from build123d import *

# Parameters (mm, degrees)
ESQUISSE1_R        = 2
ESQUISSE1_W        = 5
ESQUISSE1_H        = 10
BOSS_EXTRU_1_DEPTH = 6


with BuildPart() as part:
    # Esquisse1 → Boss.-Extru.1 (new body)
    with BuildSketch(Plane.XY):
        Polygon((0, 0), (0, 26), (-5.2, 26), (-5.2, 20), (-10, 20), (-10, 26), (-15.2, 26), (-15.2, 20), (-20, 20), (-20, 26), (-25.2, 26), (-25.2, 20), (-30, 20), (-30, 26), (-35.2, 26), (-35.2, 20), (-40, 20), (-40, 26), (-45.2, 26), (-45.2, 20), (-50, 20), (-50, 26), (-55.2, 26), (-55.2, 20), (-60, 20), (-60, 26), (-65.2, 26), (-65.2, 20), (-70, 20), (-70, 26), (-75.2, 26), (-75.2, 20), (-80, 20), (-80, 26), (-85.2, 26), (-85.2, 20), (-90, 20), (-90, 26), (-95.2, 26), (-95.2, 20), (-100, 20), (-100, 26), (-105.2, 26), (-105.2, 20), (-110, 20), (-110, 26), (-115.2, 26), (-115.2, 20), (-120, 20), (-120, 26), (-125.2, 26), (-125.2, 20), (-130, 20), (-130, 26), (-135.2, 26), (-135.2, 20), (-140, 20), (-140, 26), (-145.2, 26), (-145.2, 20), (-150, 20), (-150, 26), (-155.2, 26), (-155.2, 20), (-160, 20), (-160, 26), (-165.2, 26), (-165.2, 20), (-170, 20), (-170, 26), (-175.2, 26), (-175.2, 20), (-180, 20), (-180, 26), (-185.2, 26), (-185.2, 20), (-190, 20), (-190, 26), (-195.2, 26), (-195.2, 20), (-200, 20), (-200, 26), (-205.2, 26), (-205.2, 20), (-210, 20), (-210, 26), (-215.2, 26), (-215.2, 20), (-220, 20), (-220, 26), (-225.2, 26), (-225.2, 20), (-230, 20), (-230, 26), (-235.2, 26), (-235.2, 20), (-240, 20), (-240, 26), (-245.2, 26), (-245.2, 20), (-250, 20), (-250, 26), (-255.2, 26), (-255.2, 20), (-260, 20), (-260, 26), (-265.2, 26), (-265.2, 20), (-270, 20), (-270, 26), (-275.2, 26), (-275.2, 20), (-280, 20), (-280, 26), (-285.2, 26), (-285.2, 20), (-290, 20), (-290, 26), (-295.2, 26), (-295.2, 20), (-300, 20), (-300, 26), (-305.2, 26), (-305.2, 20), (-310, 20), (-310, 14.8), (-304, 14.8), (-304, 10), (-310, 10), (-310, 4.8), (-304, 4.8), (-304, 0), (-310, 0), (-310, -5.2), (-304, -5.2), (-304, -10), (-310, -10), (-310, -15.2), (-304, -15.2), (-304, -20), (-284, -20), (-284, 0), align=None)
        with Locations((-210, 10)):
            Circle(ESQUISSE1_R, mode=Mode.SUBTRACT)
        with Locations((-10, 10)):
            Circle(ESQUISSE1_R, mode=Mode.SUBTRACT)
        with Locations((-296.5, -5)):
            Rectangle(ESQUISSE1_W, ESQUISSE1_H, mode=Mode.SUBTRACT)
    extrude(amount=BOSS_EXTRU_1_DEPTH)


solid = part.part
Verification items for the finished model (mm, model axes). A direction names the side the tool comes from. Coordinates: 2 decimals unless noted, no trailing zeros. Write each question's results on one line, items separated by ' | '.
1) Section check A-A on y = 23. Give the number of separate pieces and of enclosed holes in the cut face, plus the area to 3 significant figures.
Solved:
separate pieces: 31 | enclosed holes: 0 | area: 967 mm²
2) Gauge pin test, flat ends, axial feed: pin 1 Ø1.4 at (y, z) = (2.5, 3.5) entering from -X; pin 2 Ø3 at (x, z) = (-257, 3.5) entering from -Y; pin 3 Ø1.4 at (x, z) = (-258, 2) entering from +Y. Record the tip position at first contact, or that the pin passes through.
Solved:
pin 1: stops at x = -304 | pin 2: stops at y = 0 | pin 3: stops at y = 20
3) Scan lines: line 1 along X through (y, z) = (-1.5, 3.6); line 2 along Y through (x, z) = (-189.5, 0.9); line 3 along Y through (x, z) = (-132, 5.25). Record each from-to range of solid material in increasing order. Write a range as [from, to].
Solved:
line 1: x = [-310, -299], [-294, -284] | line 2: y = [0, 20] | line 3: y = [0, 26]
4) Release check for a two-part mould opening along X. For faces 4 (the face through (-307, -5.2, 3)), 5 (the face through (-304, -8, 3)), 6 (the face through (-65.2, 23, 3)) record: pulls with the +X half, pulls with the -X half, needs draft (parallel to the pull), parting line crosses it, or undercut.
Solved:
face 4: needs draft | face 5: pulls with the -X half | face 6: undercut
5) Access from +Z, -Z, +X, -X, +Y, -Y to the whole of each face (thin tool, end or side, straight path). Record for faces 1 (the face through (-140, 23, 3)), 2 (the face through (-63, 26, 3)), 3 (the face through (-297, 0, 3)).
Solved:
face 1: +Z, -Z, +Y | face 2: +Z, -Z, +X, -X, +Y | face 3: +Z, -Z
